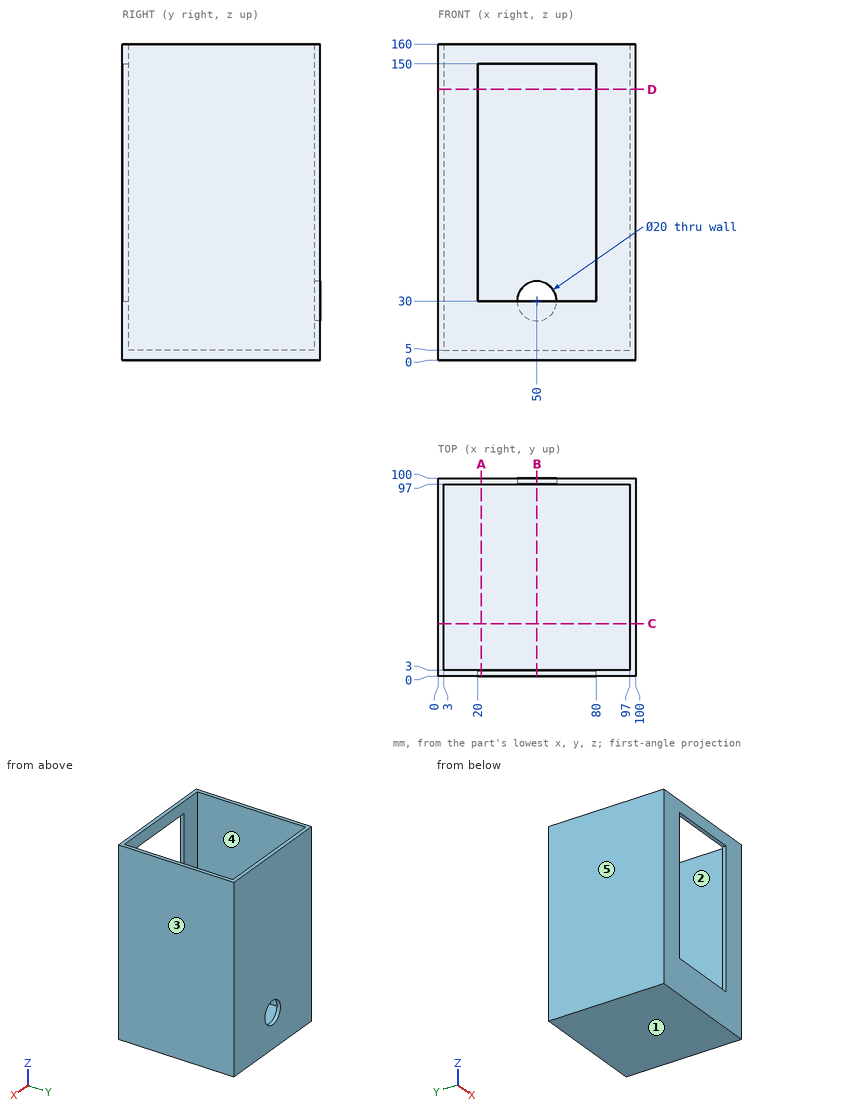
Check sheet for the drawn part. Datum: minimum x, y, z corner. Units: mm. A direction names the side the tool comes from. Give positions to 0.01 mm unless a question says otherwise; leave off trailing zeros. Write each loop counter-clockwise with the first axis right and the second up, starting at its lowest first coordinate (ties: lowest second). Pieces come first, ordered by that corner, then holes.
(1) Mould release check, pull along X, two halves, no side actions. Record for the marked faces 3, 4 and 5: +X half, -X half, draft (parallel to the pull), parting line (faces both ways), or undercut.
(2) Cross-section at B-B (x = 50). Enter the section's corners in (y, z).
(3) Cross-section at A-A (x = 22). Enter the section's corners in (y, z), plus the area to 3 significant figures.
(4) Gauge pin test, flat end, axial feed: pin 1 (12 mm diameter, centred on x = 15, y = 15, fed in from +Z). Record the tip position at first contact, or that the pin passes through.
(5) Access from +Z, -Z, +X, -X, +Y, -Y to the whole of each face (thin tool, end or side, straight path). Record for the marked faces 1 and 2.
(6) Cross-section at D-D (z = 137). Enter the section's corners in (x, y), plus the area to 3 significant figures.
(7) Cross-section at C-C (y = 26.5). Enter the section's corners in (x, z).
(8) Material ranges on line 1 (Y direction, x = 4, z = 60.5); line 2 (Z direction, x = 50, y = 99), recorded low to high.
Worked out:
1. face 3: +X half
1. face 4: undercut
1. face 5: -X half
2. outline: (0, 0) - (100, 0) - (100, 20) - (97, 20) - (97, 5) - (3, 5) - (3, 30) - (0, 30) - close; (0, 150) - (3, 150) - (3, 160) - (0, 160) - close; (97, 40) - (100, 40) - (100, 160) - (97, 160) - close
3. outline: (0, 0) - (100, 0) - (100, 160) - (97, 160) - (97, 5) - (3, 5) - (3, 30) - (0, 30) - close; (0, 150) - (3, 150) - (3, 160) - (0, 160) - close
3. area: 1,070 mm2
4. pin 1: stops at z = 5
5. face 1: -Z, +X, -X, +Y, -Y
5. face 2: +Z
6. outline: (0, 0) - (20, 0) - (20, 3) - (3, 3) - (3, 97) - (97, 97) - (97, 3) - (80, 3) - (80, 0) - (100, 0) - (100, 100) - (0, 100) - close
6. area: 984 mm2
7. outline: (0, 0) - (100, 0) - (100, 160) - (97, 160) - (97, 5) - (3, 5) - (3, 160) - (0, 160) - close
8. line 1: y = 0 to 3, 97 to 100
8. line 2: z = 0 to 20, 40 to 160
